CAD build for the part. Positions are in the model's coordinates, mm. Coordinates: 2 decimals unless noted, no trailing zeros. Loops run counter-clockwise (first coordinate to the right, second up) from the corner with the lowest first, then second, coordinate; pieces in that order, holes last. Notation, with made-up numbers: M -26.75,-40 L -20.75,-40 A23 cw -20.75,-26 Z; hole C -6.5,89.25 d4. An arc over 180 degrees is marked long. Answer as a JSON object with one key per item and string values. Group by question number.
```python
from build123d import *

# Parameters (mm, degrees)
SKETCH2_W          = 250
SKETCH2_H          = 250
BASE_DEPTH         = 3.175
SKETCH4_W          = 45.1
SKETCH4_H          = 25.1
SKETCH4_W_2        = 20.378913316
SKETCH4_H_2        = 45.1
SKETCH4_H_3        = 20.378913316
JIGSAW_DEPTH       = 10
STANDOFF_HOLES_D   = 2.5
STANDOFF_HOLES_2_D = 2.5


with BuildPart() as part:
    # Sketch2 → Base (new body)
    with BuildSketch(Plane(origin=(0, 0, 0), x_dir=(1, 0, 0), z_dir=(0, 1, 0))):
        Rectangle(SKETCH2_W, SKETCH2_H)
    extrude(amount=BASE_DEPTH)

    # Sketch4 → Jigsaw (cut)
    with BuildSketch(Plane(origin=(0, 3.175, 0), x_dir=(1, 0, 0), z_dir=(0, 1, 0))):
        with Locations((0, 125)):
            Rectangle(SKETCH4_W, SKETCH4_H)
        with Locations((-125, 0)):
            Rectangle(SKETCH4_W_2, SKETCH4_H_2)
        with Locations((125, 0)):
            Rectangle(SKETCH4_W_2, SKETCH4_H_2)
        with Locations((0, -125)):
            Rectangle(SKETCH4_W, SKETCH4_H_3)
    extrude(amount=-JIGSAW_DEPTH, mode=Mode.SUBTRACT)

    # Standoff Holes (through all)
    with Locations(Plane(origin=(0, 3.175, 0), x_dir=(1, 0, 0), z_dir=(0, 1, 0))):
        with Locations((-115, 115)):
            Hole(STANDOFF_HOLES_D / 2)

    # Standoff Holes 2 (through all)
    with Locations(Plane(origin=(0, 3.175, 0), x_dir=(1, 0, 0), z_dir=(0, 1, 0))):
        with Locations((115, 115), (115, -115), (-115, -115)):
            Hole(STANDOFF_HOLES_2_D / 2)


solid = part.part
```
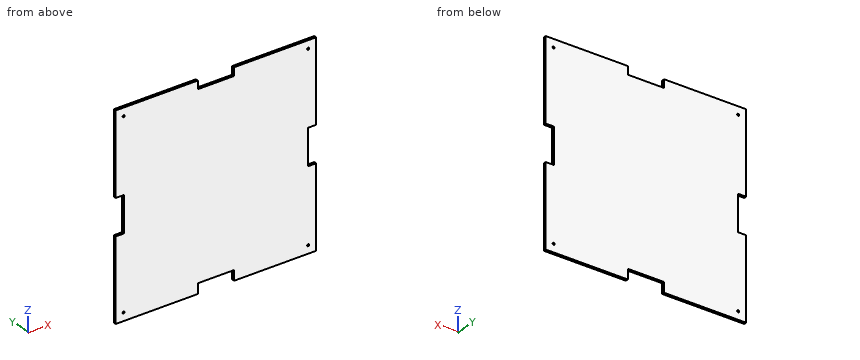
Item 1: Slice it at C-C, the plane z = 18. Write the cut outline in (x, y) (3 decimals), then the cut area to 3 significant figures.
Item 2: Drill centre lines: L1, parallel to Z at x = 115, y = 1.75; L2, parallel to Z at x = 12, y = 1.15. Where is each one in solid material? Low to high. Write a range as from..to.
Item 3: Slice it at A-A, the plane y = 0.6. Write the cut outline in (x, z), then the cut area to 3 significant figures.
Item 4: Slice it at B-B, the plane x = -13.5. Write the cut outline in (y, z) (3 decimals).
Item 5: Pin check, flat tips, straight feed: pin 1 (1 mm diameter, centred on y = 2, z = 4.5, fed in from +X); pin 2 (1.6 mm diameter, centred on x = 4, y = 1, fed in from -Z); pin 3 (3 mm diameter, centred on x = 115, z = 115, fed in from -Y); pin 4 (2 mm diameter, centred on x = -115, z = -115, fed in from -Y). Stop position of each tip, or through.
Computed:
{
 "1": {"outline": "M -114.811,0 L 114.811,0 L 114.811,3.175 L -114.811,3.175 Z", "area": "729 mm2"},
 "2": {"L1": "-125..-116.25, -113.75..-22.55, 22.55..113.75, 116.25..125", "L2": "-112.45..114.81"},
 "3": {"outline": "M -125,-125 L -22.55,-125 L -22.55,-112.45 L 22.55,-112.45 L 22.55,-125 L 125,-125 L 125,-22.55 L 114.81,-22.55 L 114.81,22.55 L 125,22.55 L 125,125 L 22.55,125 L 22.55,114.81 L -22.55,114.81 L -22.55,125 L -125,125 L -125,22.55 L -114.81,22.55 L -114.81,-22.55 L -125,-22.55 Z; hole C -115,-115 d2.5; hole C -115,115 d2.5; hole C 115,-115 d2.5; hole C 115,115 d2.5", "area": "60,500 mm2"},
 "4": {"outline": "M 0,-112.45 L 3.175,-112.45 L 3.175,114.811 L 0,114.811 Z"},
 "5": {"pin 1": "x = 114.81", "pin 2": "z = -112.45", "pin 3": "y = 0", "pin 4": "through"}
}
